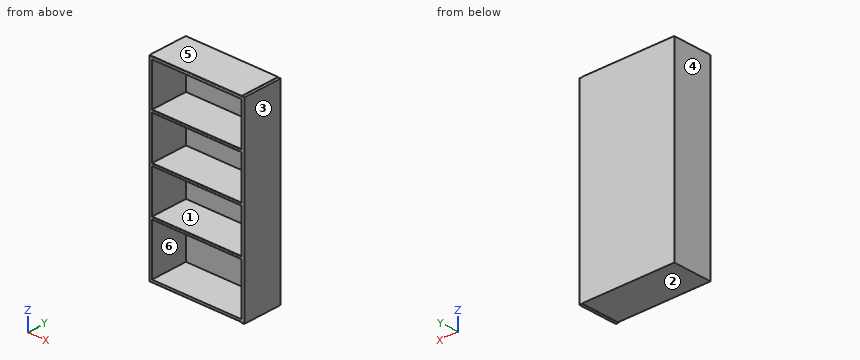
```python
from build123d import *

# Parameters (mm, degrees)
F0_W     = 863.595354099
F0_H     = 25.4
F1_DEPTH = 381
F2_R     = 5.08
F0_H_2   = 482.6
F0_H_3   = 406.4
F3_DEPTH = 25.4


with BuildPart() as f1:
    # F0 (on Front) → F1 (new body)
    with BuildSketch(Plane.XZ):
        Polygon((-12.7, 891.914858846), (-12.7, 914.4), (-12.7, 917.314858846), (-876.295354099, 917.314858846), (-876.295354099, 891.914858846), align=None)
        with Locations((-444.4976770495, -898.785141154)):
            Rectangle(F0_W, F0_H)
        Polygon((-901.695354099, -911.485141154), (-876.295354099, -911.485141154), (-876.295354099, -886.085141154), (-876.295354099, -403.485141154), (-876.295354099, -378.085141154), (-876.295354099, 28.314858846), (-876.295354099, 53.714858846), (-876.295354099, 460.114858846), (-876.295354099, 485.514858846), (-876.295354099, 891.914858846), (-876.295354099, 917.314858846), (-901.695354099, 917.314858846), align=None)
        Polygon((-12.7, -911.485141154), (-12.7, -914.4), (12.7, -914.4), (12.7, 914.4), (-12.7, 914.4), (-12.7, 891.914858846), (-12.7, 485.514858846), (-12.7, 460.114858846), (-12.7, 53.714858846), (-12.7, 28.314858846), (-12.7, -378.085141154), (-12.7, -403.485141154), (-12.7, -886.085141154), align=None)
        with Locations((-444.4976770495, 472.814858846)):
            Rectangle(F0_W, F0_H)
        with Locations((-444.4976770495, 41.014858846)):
            Rectangle(F0_W, F0_H)
        with Locations((-444.4976770495, -390.785141154)):
            Rectangle(F0_W, F0_H)
    extrude(amount=F1_DEPTH)

    # F2
    f2_edges = [f1.edges().sort_by_distance(p)[0] for p in [
        (-457.197677, -381, 917.314859),
        (-444.497677, -381, 485.514859),
        (-444.497677, -381, 460.114859),
        (-444.497677, -381, 53.714859),
        (-444.497677, -381, -378.085141),
        (-444.497677, -381, 28.314859),
        (-444.497677, -381, -403.485141),
        (-457.197677, -381, -911.485141),
    ]]
    fillet(f2_edges, radius=F2_R)

    # F0 (on Front) → F3 (join)
    with BuildSketch(Plane.XZ):
        with Locations((-444.4976770495, -644.785141154)):
            Rectangle(F0_W, F0_H_2)
        with Locations((-444.4976770495, -174.885141154)):
            Rectangle(F0_W, F0_H_3)
        with Locations((-444.4976770495, 256.914858846)):
            Rectangle(F0_W, F0_H_3)
        with Locations((-444.4976770495, 688.714858846)):
            Rectangle(F0_W, F0_H_3)
    extrude(amount=F3_DEPTH)


solid = f1.part
```
Design review of the part built by this model. Coordinates are the model's own, in mm. Face numbers are marked on the shaded views. A direction names the side the tool comes from. Round coordinates to 2 decimals unless told otherwise and drop trailing zeros. Write each loop counter-clockwise with the first axis right and the second up, starting at its lowest first coordinate (ties: lowest second). Pieces come first, ordered by that corner, then holes.
Item 1: We need section A-A on y = -235. Write out the cut boundary in (x, z), and give its area (3 significant figures).
Item 2: We need section B-B on z = -460. Write out the cut boundary in (x, y).
Item 3: For probe 1 along Z at (x, y) = (-822.5, -36.5); probe 2 along X at (y, z) = (-85, 18); probe 3 along Y at (x, z) = (-418, -798), list the stretches that pass through material, from the lowest coordinate up.
Item 4: For the marked faces 1, 2 and 3, list the 3-axis set-ups (+Z, -Z, +X, -X, +Y, -Y) from which the entire face can be reached by the end or side of a thin tool; tool diameter is ignored.
Item 5: The part is to be moulded in two halves that separate along Z. For the marked faces 4, 5 and 6, say which applies: +Z half, -Z half, draft (parallel to the pull), parting line (faces both ways), or undercut.
Item 6: Clearance check with flat-ended pins moving along their axes: pin 1 Ø1 at (x, z) = (-728, -347) entering from +Y; pin 2 Ø1.5 at (x, y) = (-597, -43.5) entering from -Z. State where each tip first meets the part, or that it passes through.
Item 7: We need section C-C on x = -338. Write out the cut boundary in (y, z), and give its area (3 significant figures).
Returned:
1. outline: (-901.7, -911.49) - (-12.7, -911.49) - (-12.7, -914.4) - (12.7, -914.4) - (12.7, 914.4) - (-12.7, 914.4) - (-12.7, 917.31) - (-901.7, 917.31) - close; hole (-876.3, -886.09) - (-12.7, -886.09) - (-12.7, -403.49) - (-876.3, -403.49) - close; hole (-876.3, -378.09) - (-12.7, -378.09) - (-12.7, 28.31) - (-876.3, 28.31) - close; hole (-876.3, 53.71) - (-12.7, 53.71) - (-12.7, 460.11) - (-876.3, 460.11) - close; hole (-876.3, 485.51) - (-12.7, 485.51) - (-12.7, 891.91) - (-876.3, 891.91) - close
1. area: 203,000 mm2
2. outline: (-901.7, -381) - (-876.3, -381) - (-876.3, -25.4) - (-12.7, -25.4) - (-12.7, -381) - (12.7, -381) - (12.7, 0) - (-901.7, 0) - close
3. probe 1: z = -911.49 to -886.09, -403.49 to -378.09, 28.31 to 53.71, 460.11 to 485.51, 891.91 to 917.31
3. probe 2: x = -901.7 to -876.3, -12.7 to 12.7
3. probe 3: y = -25.4 to 0
4. face 1: -Y
4. face 2: -Z, -X, +Y, -Y
4. face 3: +Z, -Z, +X, +Y, -Y
5. face 4: draft
5. face 5: +Z half
5. face 6: undercut
6. pin 1: stops at y = 0
6. pin 2: stops at z = -911.49
7. outline: (-381, -906.41) arc R5.08 ccw to (-375.92, -911.49) - (0, -911.49) - (0, 917.31) - (-375.92, 917.31) arc R5.08 ccw to (-381, 912.23) - (-381, 891.91) - (-25.4, 891.91) - (-25.4, 485.51) - (-375.92, 485.51) arc R5.08 ccw to (-381, 480.43) - (-381, 465.19) arc R5.08 ccw to (-375.92, 460.11) - (-25.4, 460.11) - (-25.4, 53.71) - (-375.92, 53.71) arc R5.08 ccw to (-381, 48.63) - (-381, 33.39) arc R5.08 ccw to (-375.92, 28.31) - (-25.4, 28.31) - (-25.4, -378.09) - (-375.92, -378.09) arc R5.08 ccw to (-381, -383.17) - (-381, -398.41) arc R5.08 ccw to (-375.92, -403.49) - (-25.4, -403.49) - (-25.4, -886.09) - (-381, -886.09) - close
7. area: 91,600 mm2
